Geometry: final body of the model. Coordinates: model frame, mm. A direction names the side the tool comes from. Give positions to 0.01 mm unless a question says otherwise; leave off trailing zeros. Write each loop counter-clockwise with the first axis right and the second up, starting at its lowest first coordinate (ties: lowest second). Pieces come first, ordered by that corner, then holes.
Q1. Cut plane A-A on z = -53.6. Return the cut outline in (x, y).
Q2. Cut plane B-B on y = 41. Return the cut outline in (x, z), plus the area to 4 significant figures.
Q3. Draft query along Z for faces 4 (the face through (0, 30, -46)), 5 (the face through (9, 31, -6.5)), 6 (the face through (17, 30, -90)), 7 (the face through (17, 30, 0)). Return one class per face: pulls with the +Z half, pulls with the -Z half, needs draft (parallel to the pull), parting line crosses it, or undercut.
Q4. Cut plane C-C on x = 13.5. Return the cut outline in (y, z).
Q5. Line query: L1, parallel to X at y = 12, z = -5; L2, parallel to Z at x = 33, y = 8; L3, parallel to X at y = 50.5, z = -23. Output: solid intervals per line, ascending.
Q6. Reachability of faces 1 (the face through (17, -3, -44)), 2 (the face through (9, 31, -83.5)), 3 (the face through (32.52, 9.11, -52.49)) from +Z, -Z, +X, -X, +Y, -Y: full face, straight path, thin tool, end or side. Return the list, or none.
Q7. Cut plane D-D on y = 8.1. Return the cut outline in (x, z).
```python
from build123d import *

# Parameters (mm, degrees)
ESBO_O1_W                = 34
ESBO_O1_H                = 90
RESSALTO_EXTRUS_O1_DEPTH = 63
ESBO_O2_W                = 34
ESBO_O2_H                = 90
RESSALTO_EXTRUS_O2_DEPTH = 3
ESBO_O3_R                = 1.5
CORTE_EXTRUS_O1_DEPTH    = 3


with BuildPart() as part:
    # Esboço1 → Ressalto-extrusão1 (new body)
    with BuildSketch(Plane(origin=(0, 0, 0), x_dir=(1, 0, 0), z_dir=(0, 1, 0))):
        with Locations((17, 45)):
            Rectangle(ESBO_O1_W, ESBO_O1_H)
        Polygon((5.5, 8), (3, 8), (3, 82), (5.5, 82), (5.5, 87), (7.7, 87), (7.7, 83.5), (10.2, 83.5), (10.2, 87), (31, 87), (31, 3), (10.2, 3), (10.2, 6.5), (7.7, 6.5), (7.7, 3), (5.5, 3), align=None, mode=Mode.SUBTRACT)
    extrude(amount=RESSALTO_EXTRUS_O1_DEPTH)

    # Esboço2 → Ressalto-extrusão2 (add)
    with BuildSketch(Plane.XZ):
        with Locations((17, -45)):
            Rectangle(ESBO_O2_W, ESBO_O2_H)
    extrude(amount=RESSALTO_EXTRUS_O2_DEPTH)

    # Esboço3 → Corte-extrusão1 (cut)
    with BuildSketch(Plane(origin=(34, 0, 0), x_dir=(0, 0, -1), z_dir=(1, 0, 0))):
        with Locations((53.6, 8.1)):
            Circle(ESBO_O3_R)
    extrude(amount=-CORTE_EXTRUS_O1_DEPTH, mode=Mode.SUBTRACT)


solid = part.part
```
Data:
1. outline: (0, -3) - (34, -3) - (34, 6.6) - (31, 6.6) - (31, 0) - (3, 0) - (3, 63) - (0, 63) - close; (31, 9.6) - (34, 9.6) - (34, 63) - (31, 63) - close
2. outline: (0, -90) - (34, -90) - (34, 0) - (0, 0) - close; hole (3, -82) - (5.5, -82) - (5.5, -87) - (7.7, -87) - (7.7, -83.5) - (10.2, -83.5) - (10.2, -87) - (31, -87) - (31, -3) - (10.2, -3) - (10.2, -6.5) - (7.7, -6.5) - (7.7, -3) - (5.5, -3) - (5.5, -8) - (3, -8) - close
2. area: 750.5 mm2
3. face 4: needs draft
3. face 5: undercut
3. face 6: pulls with the -Z half
3. face 7: pulls with the +Z half
4. outline: (-3, -90) - (63, -90) - (63, -87) - (0, -87) - (0, -3) - (63, -3) - (63, 0) - (-3, 0) - close
5. L1: x = 0 to 5.5, 7.7 to 10.2, 31 to 34
5. L2: z = -90 to -55.1, -52.1 to 0
5. L3: x = 0 to 3, 31 to 34
6. face 1: +Z, -Z, +X, -X, -Y
6. face 2: +Y
6. face 3: +X
7. outline: (0, -90) - (34, -90) - (34, -55.1) - (31, -55.1) - (31, -87) - (10.2, -87) - (10.2, -83.5) - (7.7, -83.5) - (7.7, -87) - (5.5, -87) - (5.5, -82) - (3, -82) - (3, -8) - (5.5, -8) - (5.5, -3) - (7.7, -3) - (7.7, -6.5) - (10.2, -6.5) - (10.2, -3) - (31, -3) - (31, -52.1) - (34, -52.1) - (34, 0) - (0, 0) - close
